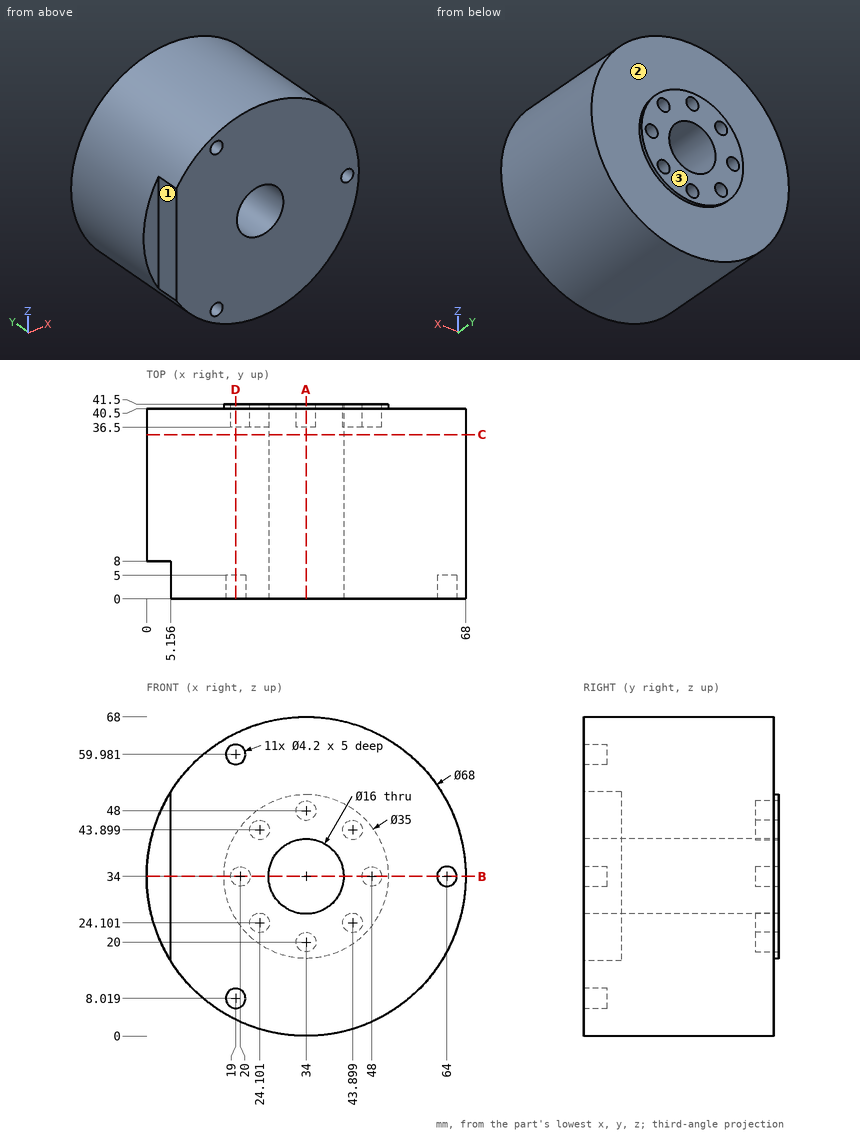
Input: dimensioned drawing with shaded views. Units: mm. Origin: part minimum x, y, z. A direction names the side the tool comes from. Coordinates: 2 decimals unless noted, no trailing zeros. Order: outer loops, then holes, each group sorted by start corner. A loop starts at its lowest first (then second) coordinate and runs counter-clockwise, first axis right, second up. Notation, with made-up numbers: (19.25, 62) - (30.25, 62) arc R22 cw to (30.25, 97) - close; hole circle Ø3 at (65, 14.5). An arc over 180 degrees is marked (long way). Return JSON: item names as keys, results as strings. Group by question number.
1. Cut plane A-A (x = 34). Output: boundary loops of the cut face in (y, z).
2. Cut plane C-C (y = 35). Output: boundary loops of the cut face in (x, z).
3. Cut plane D-D (x = 19). Output: boundary loops of the cut face in (y, z).
4. Set-up query: the marked faces 1, 2 and 3. Return all of +Z, -Z, +X, -X, +Y, -Y with unobstructed straight access to the full face (end or side cutting, diameter ignored); none if empty.
5. Pin query (flat end, axial travel): pin 1 (12 mm diameter, centred on x = 55.5, z = 9.5, fed in from +Y); pin 2 (2 mm diameter, centred on x = 63.5, z = 34.5, fed in from -Y); pin 3 (1.5 mm diameter, centred on y = 29.5, z = 32, fed in from -X). Return the tip coordinate at first contact, or that it passes through.
6. Cut plane B-B (z = 34). Output: boundary loops of the cut face in (x, y) (1 decimal), plus the area to 3 significant figures.
7. Material intervals for line 1 along X through (y, z) = (40.1, 34); line 2 along X through (y, z) = (1, 34) (1 decimal); line 3 along Y through (x, z) = (35, 63), sorted ascending. Write a range as [from, to].
Resolved:
{
 "1": {"outline": "(0, 0) - (40.5, 0) - (40.5, 16.5) - (41.5, 16.5) - (41.5, 17.9) - (36.5, 17.9) - (36.5, 22.1) - (41.5, 22.1) - (41.5, 26) - (0, 26) - close; (0, 42) - (41.5, 42) - (41.5, 45.9) - (36.5, 45.9) - (36.5, 50.1) - (41.5, 50.1) - (41.5, 51.5) - (40.5, 51.5) - (40.5, 68) - (0, 68) - close"},
 "2": {"outline": "circle Ø68 at (34, 34); hole circle Ø16 at (34, 34)"},
 "3": {"outline": "(0, 3.49) - (40.5, 3.49) - (40.5, 24.99) - (41.5, 24.99) - (41.5, 32.15) - (36.5, 32.15) - (36.5, 35.85) - (41.5, 35.85) - (41.5, 43.01) - (40.5, 43.01) - (40.5, 64.51) - (0, 64.51) - (0, 62.08) - (5, 62.08) - (5, 57.88) - (0, 57.88) - (0, 10.12) - (5, 10.12) - (5, 5.92) - (0, 5.92) - close"},
 "4": {"face 1": "+Z, -Z, -X, -Y", "face 2": "+Y", "face 3": "+Z, -Z, +X, -X, +Y"},
 "5": {"pin 1": "stops at y = 40.5", "pin 2": "stops at y = 5", "pin 3": "stops at x = 0.02"},
 "6": {"outline": "(0, 8) - (5.2, 8) - (5.2, 0) - (26, 0) - (26, 41.5) - (22.1, 41.5) - (22.1, 36.5) - (17.9, 36.5) - (17.9, 41.5) - (16.5, 41.5) - (16.5, 40.5) - (0, 40.5) - close; (42, 0) - (61.9, 0) - (61.9, 5) - (66.1, 5) - (66.1, 0) - (68, 0) - (68, 40.5) - (51.5, 40.5) - (51.5, 41.5) - (50.1, 41.5) - (50.1, 36.5) - (45.9, 36.5) - (45.9, 41.5) - (42, 41.5) - close", "area": "2,020 mm²"},
 "7": {"line 1": "x = [0, 17.9], [22.1, 26], [42, 45.9], [50.1, 68]", "line 2": "x = [5.2, 26], [42, 61.9], [66.1, 68]", "line 3": "y = [0, 40.5]"}
}
